```python
from build123d import *

# Parameters (mm, degrees)
SKETCH1_W                                        = 185
SKETCH1_H                                        = 55
BOSS_EXTRUDE1_DEPTH                              = 49
BOSS_EXTRUDE2_DEPTH                              = 10
SKETCH4_W                                        = 57.5
SKETCH4_H                                        = 15
CUT_EXTRUDE2_DEPTH                               = 66
SKETCH5_W                                        = 57.5
SKETCH5_H                                        = 15
CUT_EXTRUDE3_DEPTH                               = 56
BOSS_EXTRUDE3_DEPTH                              = 10
BOSS_EXTRUDE4_DEPTH                              = 3.5
BOSS_EXTRUDE7_DEPTH                              = 3.5
BOSS_EXTRUDE8_DEPTH                              = 3.5
SKETCH14_W                                       = 70
SKETCH14_H                                       = 4.263818571
CUT_EXTRUDE5_DEPTH                               = 59.5
SKETCH15_W                                       = 57.5
SKETCH15_H                                       = 34
BOSS_EXTRUDE9_DEPTH                              = 20
CBORE_FOR_M4_PAN_HEAD_MACHINE_SCREW1_D           = 4.5
CBORE_FOR_M4_PAN_HEAD_MACHINE_SCREW1_CBORE_D     = 9
CBORE_FOR_M4_PAN_HEAD_MACHINE_SCREW1_CBORE_DEPTH = 3.1
SKETCH19_W                                       = 70
SKETCH19_H                                       = 8.146045787
BOSS_EXTRUDE10_DEPTH                             = 34.74
SKETCH20_W                                       = 18
SKETCH20_H                                       = 6.271934352
BOSS_EXTRUDE11_DEPTH                             = 15
FILLET1_R                                        = 5
SKETCH21_R                                       = 11.25
CUT_EXTRUDE6_DEPTH                               = 80.476181429
FILLET2_R                                        = 5


with BuildPart() as part:
    # Sketch1 → Boss-Extrude1 (new body)
    with BuildSketch(Plane.XZ.offset(15)):
        with Locations((0, 27.5)):
            Rectangle(SKETCH1_W, SKETCH1_H)
    extrude(amount=-BOSS_EXTRUDE1_DEPTH)

    # Sketch2 → Boss-Extrude2 (add)
    with BuildSketch(Plane.XY.offset(55)):
        with BuildLine():
            Line((26.525, -10.2), (3.725, -10.2))
            ThreePointArc((3.725, -10.2), (2.375, -8.85), (3.725, -7.5))
            Line((3.725, -7.5), (26.525, -7.5))
            ThreePointArc((26.525, -7.5), (27.875, -8.85), (26.525, -10.2))
        make_face()
    extrude(amount=BOSS_EXTRUDE2_DEPTH)

    # Sketch4 → Cut-Extrude2 (cut, through all)
    with BuildSketch(Plane(origin=(0, 0, 0), x_dir=(-1, 0, 0), z_dir=(0, 0, -1))):
        with Locations((-63.75, -7.5)):
            Rectangle(SKETCH4_W, SKETCH4_H)
    extrude(amount=-CUT_EXTRUDE2_DEPTH, mode=Mode.SUBTRACT)

    # Sketch5 → Cut-Extrude3 (cut, through all)
    with BuildSketch(Plane.XY.offset(55)):
        with Locations((-63.75, -7.5)):
            Rectangle(SKETCH5_W, SKETCH5_H)
    extrude(amount=-CUT_EXTRUDE3_DEPTH, mode=Mode.SUBTRACT)

    # Sketch6 → Boss-Extrude3 (add)
    with BuildSketch(Plane.XY.offset(55)):
        with BuildLine():
            Line((-26.525, -7.5), (-3.725, -7.5))
            ThreePointArc((-3.725, -7.5), (-2.375, -8.85), (-3.725, -10.2))
            Line((-3.725, -10.2), (-26.525, -10.2))
            ThreePointArc((-26.525, -10.2), (-27.875, -8.85), (-26.525, -7.5))
        make_face()
    extrude(amount=BOSS_EXTRUDE3_DEPTH)

    # Sketch8 → Boss-Extrude4 (add)
    with BuildSketch(Plane(origin=(0, 0, 0), x_dir=(-1, 0, 0), z_dir=(0, 0, -1))):
        with BuildLine():
            Line((-11.45, 16.55), (11.45, 16.55))
            ThreePointArc((11.45, 16.55), (12.75, 15.25), (11.45, 13.95))
            Line((11.45, 13.95), (-11.45, 13.95))
            ThreePointArc((-11.45, 13.95), (-12.75, 15.25), (-11.45, 16.55))
        make_face()
    extrude(amount=BOSS_EXTRUDE4_DEPTH)

    # Sketch11 → Boss-Extrude7 (add)
    with BuildSketch(Plane(origin=(0, 0, 0), x_dir=(-1, 0, 0), z_dir=(0, 0, -1))):
        with BuildLine():
            Line((-31, -3), (31, -3))
            ThreePointArc((31, -3), (33.25, -5.25), (31, -7.5))
            Line((31, -7.5), (-31, -7.5))
            ThreePointArc((-31, -7.5), (-33.25, -5.25), (-31, -3))
        make_face()
    extrude(amount=BOSS_EXTRUDE7_DEPTH)

    # Sketch10 → Boss-Extrude8 (add)
    with BuildSketch(Plane(origin=(0, 0, 0), x_dir=(-1, 0, 0), z_dir=(0, 0, -1))):
        with BuildLine():
            Line((-18.55, 13.95), (-42.45, 13.95))
            ThreePointArc((-42.45, 13.95), (-43.75, 15.25), (-42.45, 16.55))
            Line((-42.45, 16.55), (-18.55, 16.55))
            ThreePointArc((-18.55, 16.55), (-17.25, 15.25), (-18.55, 13.95))
        make_face()
        with BuildLine():
            Line((42.45, 16.55), (18.55, 16.55))
            ThreePointArc((18.55, 16.55), (17.25, 15.25), (18.55, 13.95))
            Line((18.55, 13.95), (42.45, 13.95))
            ThreePointArc((42.45, 13.95), (43.75, 15.25), (42.45, 16.55))
        make_face()
    extrude(amount=BOSS_EXTRUDE8_DEPTH)

    # Sketch14 → Cut-Extrude5 (cut, through all)
    with BuildSketch(Plane.XY.offset(55)):
        with Locations((0, -12.868090715)):
            Rectangle(SKETCH14_W, SKETCH14_H)
    extrude(amount=-CUT_EXTRUDE5_DEPTH, mode=Mode.SUBTRACT)

    # Sketch15 → Boss-Extrude9 (add)
    with BuildSketch(Plane.XY.offset(55)):
        with Locations((-63.75, 17)):
            Rectangle(SKETCH15_W, SKETCH15_H)
        with Locations((63.75, 17)):
            Rectangle(SKETCH15_W, SKETCH15_H)
    extrude(amount=BOSS_EXTRUDE9_DEPTH)

    # CBORE for M4 Pan Head Machine Screw1 (through all)
    with Locations(Plane.XZ):
        with Locations((-55.5, 63.5), (-83.5, 63.5), (-83.5, 36), (-55.5, 36), (55.5, 36), (83.5, 36), (83.5, 63.5), (55.5, 63.5)):
            CounterBoreHole(CBORE_FOR_M4_PAN_HEAD_MACHINE_SCREW1_D / 2, CBORE_FOR_M4_PAN_HEAD_MACHINE_SCREW1_CBORE_D / 2, CBORE_FOR_M4_PAN_HEAD_MACHINE_SCREW1_CBORE_DEPTH)

    # Sketch19 → Boss-Extrude10 (add)
    with BuildSketch(Plane.XZ.offset(10.736181429)):
        with Locations((0, 50.926977107)):
            Rectangle(SKETCH19_W, SKETCH19_H)
    extrude(amount=BOSS_EXTRUDE10_DEPTH)

    # Sketch20 → Boss-Extrude11 (add)
    with BuildSketch(Plane.XY.offset(55)):
        with Locations((0, -42.335967176)):
            Rectangle(SKETCH20_W, SKETCH20_H)
    extrude(amount=BOSS_EXTRUDE11_DEPTH)

    # Fillet1
    fillet1_edges = [part.edges().sort_by_distance(p)[0] for p in [
        (-92.5, 17, 75),
        (92.5, 17, 75),
        (0, -45.476181429, 46.853954213),
        (92.5, 17, 0),
        (-92.5, 17, 0),
    ]]
    fillet(fillet1_edges, radius=FILLET1_R)

    # Sketch21 → Cut-Extrude6 (cut, through all)
    with BuildSketch(Plane(origin=(0, 34, 0), x_dir=(1, 0, 0), z_dir=(0, 1, 0))):
        with Locations((0, -25.818049532)):
            Circle(SKETCH21_R)
    extrude(amount=-CUT_EXTRUDE6_DEPTH, mode=Mode.SUBTRACT)

    # Fillet2
    fillet2_edges = [part.edges().sort_by_distance(p)[0] for p in [
        (-11.25, 34, 25.818049532),
    ]]
    fillet(fillet2_edges, radius=FILLET2_R)


solid = part.part
```
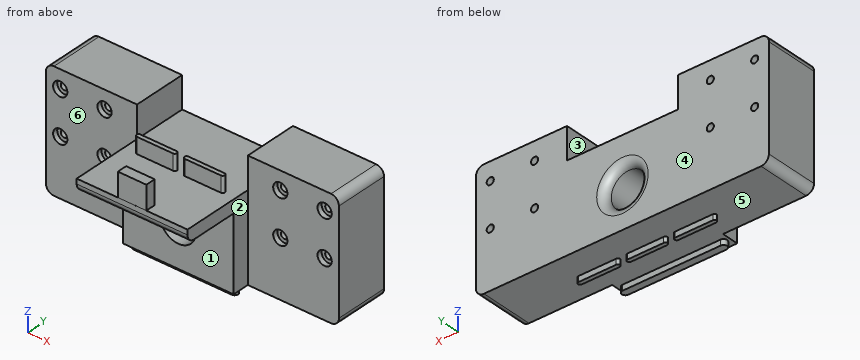
The listing builds one solid part. Answer for the finished solid, in the listing's coordinates (mm). Face numbers are marked on the shaded views. A direction names the side the tool comes from. Give positions to 0.01 mm unless a question says otherwise; leave off trailing zeros. Write each loop counter-clockwise with the first axis right and the second up, starting at its lowest first coordinate (ties: lowest second). Pieces come first, ordered by that corner, then holes. Notation, with made-up numbers: (8.25, 50.25) - (18.25, 50.25) arc R21 cw to (18.25, 56.25) - close; hole circle Ø11 at (53.5, -2). An arc over 180 degrees is marked (long way). Use one line per item in the form item = value. Start each with the question number.
1) Flat-ended cylindrical pins translate along their axes: pin 1 Ø1.8 at (x, z) = (-34.5, -1.5) entering from +Y; pin 2 Ø12 at (x, y) = (13, 8) entering from -Z; pin 3 Ø1 at (x, z) = (26.5, -1) entering from -Y. Find the tip coordinate at first contact, or state that the pin passes through.
2) Consider line 1 along Z through (x, y) = (83.5, 26); line 2 along Z through (x, y) = (-83.5, 2.3); line 3 along Y through (x, z) = (-65, 6). Determine where each line is inside the solid, lowest interval first. Write a range as from..to.
3) Find section C-C on y = -22.5. Determine the outline of the cut face in (x, z).
4) Find section B-B on y = 19. Count the separate pieces of the cut face and the enclosed holes in it, plus the area to 3 significant figures.
5) A tool of negligible diameter and unlimited length cuts with its end or side. For the marked faces 1, 2 and 3, from which of +Z, -Z, +X, -X, +Y, -Y can it reach the whole face along a straight path? Write none if from no direction.
6) The mould has two halves that part along Y. Classify the marked faces 4, 5 and 6: pulls with the +Y half, pulls with the -Y half, needs draft (parallel to the pull), parting line crosses it, or undercut.
7) Find section A-A on x = -83.5. Determine the outline of the cut face in (y, z).
Geometry results:
q1.pin_1 = 16.55
q1.pin_2 = 0
q1.pin_3 = -7.5
q2.line_1 = 0..33.75, 38.25..61.25, 65.75..75
q2.line_2 = 0..31.5, 40.5..59, 68..75
q2.line_3 = 0..34
q3.outline = (-35, 46.85) - (35, 46.85) - (35, 55) - (-35, 55) - close
q4.separate_pieces = 1
q4.enclosed_holes = 9
q4.area = 11,900 mm2
q5.face_1 = -Z, +X, -X, -Y
q5.face_2 = +Z, -Z, +X, -Y
q5.face_3 = +Z, +Y, -Y
q6.face_4 = pulls with the +Y half
q6.face_5 = undercut
q6.face_6 = pulls with the -Y half
q7.outline = (0, 0) - (34, 0) - (34, 33.75) - (3.1, 33.75) - (3.1, 31.5) - (0, 31.5) - close; (0, 40.5) - (3.1, 40.5) - (3.1, 38.25) - (34, 38.25) - (34, 61.25) - (3.1, 61.25) - (3.1, 59) - (0, 59) - close; (0, 68) - (3.1, 68) - (3.1, 65.75) - (34, 65.75) - (34, 75) - (0, 75) - close
